The figure shows three views and two pictorial views of one solid part (mm, origin at its lowest corner). Answer the questions. Coordinates: 2 decimals unless noted, no trailing zeros. Order: outer loops, then holes, each group sorted by start corner. A loop starts at its lowest first (then second) coordinate and runs counter-clockwise, first axis right, second up. Notation, with made-up numbers: M 77,51.25 L 123,51.25 A12 cw 123,68.25 Z; hole C 83,32.25 d3. An arc over 180 degrees is marked long. Answer in a Markdown table with one row per item. Add a question column.
Item 1: The part is cut by section B-B (z = 5). Write down the section's boundary in (x, y) (1 decimal), then the cut area to 3 significant figures.
Item 2: The part is cut by section D-D (x = 17). Write down the section's boundary in (y, z).
Item 3: The part is cut by section A-A (y = 1.05). State how many separate pieces and enclosed holes the cut face has, then the cut area to 3 significant figures.
Item 4: The part is cut by section C-C (x = 9). Write down the section's boundary in (y, z) (1 decimal).
Item 5: Consider line 1 (Z direction, x = 57, y = 0.3) (1 decimal); line 2 (X direction, y = 1.5, z = 9); line 3 (Z direction, x = 4.5, y = 0.15). Determine where each line is inside the solid, lowest interval first. Write a range as from..to.
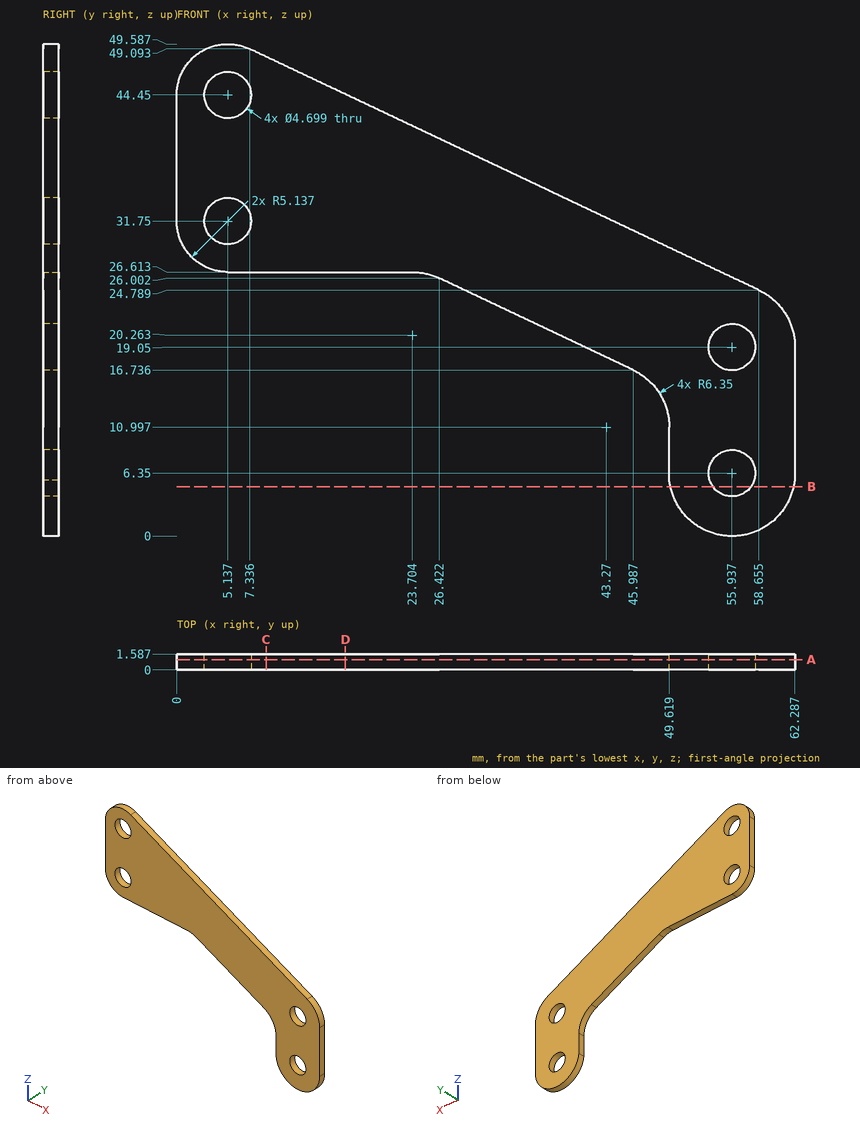
Reply:
| question | item | result |
|---|---|---|
| 1 | outline | M 49.7,0 L 54,0 L 54,1.6 L 49.7,1.6 Z; M 57.9,0 L 62.1,0 L 62.1,1.6 L 57.9,1.6 Z |
| 1 | area | 13.6 mm2 |
| 2 | outline | M 0,26.61 L 1.59,26.61 L 1.59,44.52 L 0,44.52 Z |
| 3 | separate pieces | 1 |
| 3 | enclosed holes | 4 |
| 3 | area | 1,070 mm2 |
| 4 | outline | M 0,26.6 L 1.6,26.6 L 1.6,48.3 L 0,48.3 Z |
| 5 | line 1 | z = 0.1..4.3, 8.4..17, 21.1..25.6 |
| 5 | line 2 | x = 49.62..62.29 |
| 5 | line 3 | z = 26.65..29.49, 34.01..42.19, 46.71..49.55 |
